```python
from build123d import *

# Parameters (mm, degrees)
SKETCH_W         = 105
SKETCH_H         = 28.7
PAD_DEPTH        = 2
FILLET_R         = 2.5
HOLE_D           = 3.2
HOLE_DEPTH       = 25
HOLE_CSINK_D     = 6.8
HOLE_CSINK_ANGLE = 90


with BuildPart() as part:
    # Sketch → Pad (new body)
    with BuildSketch(Plane.XZ):
        Rectangle(SKETCH_W, SKETCH_H)
    extrude(amount=-PAD_DEPTH)

    # Fillet
    fillet_edges = [part.edges().sort_by_distance(p)[0] for p in [
        (52.5, 1, 14.35),
        (52.5, 1, -14.35),
        (-52.5, 1, 14.35),
        (-52.5, 1, -14.35),
    ]]
    fillet(fillet_edges, radius=FILLET_R)

    # Hole
    with Locations(Plane.XZ):
        with Locations((46.5, 10.85), (46.5, -10.85), (-46.5, -10.85), (-46.5, 10.85)):
            CounterSinkHole(HOLE_D / 2, HOLE_CSINK_D / 2, depth=HOLE_DEPTH, counter_sink_angle=HOLE_CSINK_ANGLE)


solid = part.part
```
Model file for the job. Use its own axes, mm. Coordinates: 2 decimals unless noted, no trailing zeros. Write each loop counter-clockwise with the first axis right and the second up, starting at its lowest first coordinate (ties: lowest second). Pieces come first, ordered by that corner, then holes. Notation, with made-up numbers: (66.5, 40) - (99.5, 40) arc R29 ccw to (99.5, 79) - close; hole circle Ø6 at (-12.75, 2). An arc over 180 degrees is marked (long way). Use a Markdown table: item, result. Add a question column.
Item 1: Band-saw the part on B-B, the plane y = 0.6. Write the cut outline in (x, z), and give its area (3 significant figures).
Item 2: Band-saw the part on A-A, the plane x = -46.5. Write the cut outline in (y, z).
Item 3: Drill centre lines: line 1 along Z through (x, y) = (46.5, 1.9); line 2 along X through (y, z) = (1.9, -10.85); line 3 along X through (y, z) = (1.85, 13.25). Where is each one in solid material? Low to high.
Item 4: Band-saw the part on C-C, the plane z = 10.85. Write the cut outline in (x, y), and give its area (3 significant figures).
Item 5: Drop flat-ended pins along their axis: pin 1 (1.5 mm diameter, centred on x = 30, z = -1, fed in from -Y); pin 2 (3.5 mm diameter, centred on x = -46.5, z = 10.85, fed in from -Y). Give the stop position or say it passes through.
A:
| question | item | result |
|---|---|---|
| 1 | outline | (-52.5, -11.85) arc R2.5 ccw to (-50, -14.35) - (50, -14.35) arc R2.5 ccw to (52.5, -11.85) - (52.5, 11.85) arc R2.5 ccw to (50, 14.35) - (-50, 14.35) arc R2.5 ccw to (-52.5, 11.85) - close; hole circle Ø5.6 at (-46.5, -10.85); hole circle Ø5.6 at (-46.5, 10.85); hole circle Ø5.6 at (46.5, -10.85); hole circle Ø5.6 at (46.5, 10.85) |
| 1 | area | 2,910 mm² |
| 2 | outline | (0, -14.35) - (2, -14.35) - (2, -12.45) - (1.8, -12.45) - (0, -14.25) - close; (0, -7.45) - (1.8, -9.25) - (2, -9.25) - (2, 9.25) - (1.8, 9.25) - (0, 7.45) - close; (0, 14.25) - (1.8, 12.45) - (2, 12.45) - (2, 14.35) - (0, 14.35) - close |
| 3 | line 1 | z = -14.35 to -12.45, -9.25 to 9.25, 12.45 to 14.35 |
| 3 | line 2 | x = -52.5 to -48.1, -44.9 to 44.9, 48.1 to 52.5 |
| 3 | line 3 | x = -52.07 to 52.07 |
| 4 | outline | (-52.5, 0) - (-49.9, 0) - (-48.1, 1.8) - (-48.1, 2) - (-52.5, 2) - close; (-44.9, 1.8) - (-43.1, 0) - (43.1, 0) - (44.9, 1.8) - (44.9, 2) - (-44.9, 2) - close; (48.1, 1.8) - (49.9, 0) - (52.5, 0) - (52.5, 2) - (48.1, 2) - close |
| 4 | area | 191 mm² |
| 5 | pin 1 | stops at y = 0 |
| 5 | pin 2 | stops at y = 1.65 |
